The listing builds one solid part. Answer for the finished solid, in the listing's coordinates (mm). Give positions to 0.01 mm unless a question says otherwise; leave off trailing zeros. Order: outer loops, then holes, each group sorted by start corner. A loop starts at its lowest first (then second) coordinate and runs counter-clockwise, first axis right, second up. Notation, with made-up numbers: (61.25, 69) - (103.25, 69) arc R30 ccw to (103.25, 105) - close; hole circle Ø5 at (14, 9.25). An arc over 180 degrees is marked (long way). Use a Markdown table: item, result. Add a question column.
1) Find section A-A, the plane x = 0. Determine the outline of the cut face in (y, z), plus the area to 3 significant figures.
2) Find section D-D, the plane z = 146. Determine the outline of the cut face in (x, y).
3) Flat-ended cylindrical pins translate along their axes: pin 1 (1.5 mm diameter, centred on y = 1.5, z = 44.5, fed in from -X); pin 2 (3 mm diameter, centred on x = 4, z = 46, fed in from +Y). Find the tip coordinate at first contact, or state that the pin passes through.
4) Straight lines are drawn through the part: line 1 (Y direction, x = 0, z = 3.5); line 2 (Z direction, x = -0.75, y = 3); line 3 (Z direction, x = 4.75, y = -0.75). For each, find the intervals that lie inside material, in ascending order.
5) Find section C-C, the plane z = 25. Determine the outline of the cut face in (x, y), plus the area to 3 significant figures.
from build123d import *

# Parameters (mm, degrees)
F0_R      = 5.2451
F1_DEPTH  = 53.5432
F2_R      = 4.191
F3_DEPTH  = 6.35
F4_R      = 4.370917
F5_DEPTH  = 53.5432
F6_R      = 3.65125
F7_DEPTH  = 53.5432
F8_R      = 3.048
F9_DEPTH  = 53.5432
F10_R     = 2.54
F11_DEPTH = 53.5432


with BuildPart() as f1:
    # F0 (on Top) → F1 (new body)
    with BuildSketch(Plane.XY):
        Circle(F0_R)
    extrude(amount=F1_DEPTH)

    # F2 (on face) → F3 (cut)
    with BuildSketch(Plane(origin=(0, 0, 0), x_dir=(1, 0, 0), z_dir=(0, 0, -1))):
        Circle(F2_R)
    extrude(amount=-F3_DEPTH, mode=Mode.SUBTRACT)

    # F4 (on face) → F5 (join)
    with BuildSketch(Plane.XY.offset(53.5432)):
        Circle(F4_R)
    extrude(amount=F5_DEPTH)

    # F6 (on face) → F7 (join)
    with BuildSketch(Plane.XY.offset(107.0864)):
        Circle(F6_R)
    extrude(amount=F7_DEPTH)

    # F8 (on face) → F9 (join)
    with BuildSketch(Plane.XY.offset(160.6296)):
        Circle(F8_R)
    extrude(amount=F9_DEPTH)

    # F10 (on face) → F11 (join)
    with BuildSketch(Plane.XY.offset(214.1728)):
        Circle(F10_R)
    extrude(amount=F11_DEPTH)


solid = f1.part
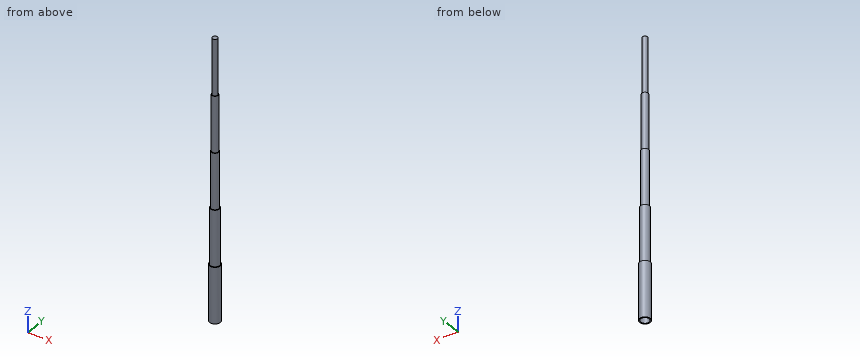
The answers:
| question | item | result |
|---|---|---|
| 1 | outline | (-5.25, 0) - (-4.19, 0) - (-4.19, 6.35) - (4.19, 6.35) - (4.19, 0) - (5.25, 0) - (5.25, 53.54) - (4.37, 53.54) - (4.37, 107.09) - (3.65, 107.09) - (3.65, 160.63) - (3.05, 160.63) - (3.05, 214.17) - (2.54, 214.17) - (2.54, 267.72) - (-2.54, 267.72) - (-2.54, 214.17) - (-3.05, 214.17) - (-3.05, 160.63) - (-3.65, 160.63) - (-3.65, 107.09) - (-4.37, 107.09) - (-4.37, 53.54) - (-5.25, 53.54) - close |
| 1 | area | 1,970 mm2 |
| 2 | outline | circle Ø7.3 at (0, 0) |
| 3 | pin 1 | x = -5.19 |
| 3 | pin 2 | y = 4.61 |
| 4 | line 1 | -5.25 to -4.19, 4.19 to 5.25 |
| 4 | line 2 | 6.35 to 160.63 |
| 4 | line 3 | 0 to 53.54 |
| 5 | outline | circle Ø10.49 at (0, 0) |
| 5 | area | 86.4 mm2 |
